```python
from build123d import *

# Parameters (mm, degrees)
F2_R = 8.554368
F3_R = 0.645964
F4_R = 0.880727
F5_R = 1.452178


with BuildPart() as f1:
    # F0 (on Front) → F1 (revolve)
    with BuildSketch(Plane.XZ):
        Polygon((-7.7875, 0), (0, 0), (0, 18.112501), (-0.9625, 18.112501), (-3.4125, 16.887501), (-6.0375, 12.1625), (-4.9875, 10.4125), (-6.0375, 10.2375), align=None)
    revolve(axis=Axis((0, 0, 9.056251), (0, 0, -1)))

    # F2
    f2_edges = [f1.edges().sort_by_distance(p)[0] for p in [
        (3.4125, 0, 16.887501),
    ]]
    fillet(f2_edges, radius=F2_R)

    # F3
    f3_edges = [f1.edges().sort_by_distance(p)[0] for p in [
        (6.0375, 0, 12.1625),
    ]]
    fillet(f3_edges, radius=F3_R)

    # F4
    f4_edges = [f1.edges().sort_by_distance(p)[0] for p in [
        (6.0375, 0, 10.2375),
    ]]
    fillet(f4_edges, radius=F4_R)

    # F5
    f5_edges = [f1.edges().sort_by_distance(p)[0] for p in [
        (7.7875, 0, 0),
    ]]
    fillet(f5_edges, radius=F5_R)


solid = f1.part
```
Check sheet for the modelled part. Datum: model origin and axes. Units: mm. Coordinates: 2 decimals unless noted, no trailing zeros. Loops run counter-clockwise (first coordinate to the right, second up) from the corner with the lowest first, then second, coordinate; pieces in that order, holes last.
1) Sectioned sample at A-A (z = 6). Record the boundary of the cut face in (x, y), and give its area (3 significant figures).
2) Gauge pin test, flat ends, axial feed: pin 1 (4 mm diameter, centred on x = -3.5, z = 9.5, fed in from +Y); pin 2 (5 mm diameter, centred on x = 1.5, z = 7, fed in from -Y); pin 3 (1.5 mm diameter, centred on x = 6, z = 9, fed in from +Y). Record the tip position at first contact, or that the pin passes through.
3) Sectioned sample at B-B (z = 9). Record the boundary of the cut face in (x, y), and give its area (3 significant figures).
4) Material ranges on probe 1 along X at (y, z) = (5.25, 1.5); probe 2 along Z at (x, y) = (-0.75, -2); probe 3 along X at (y, z) = (5.75, 5.25), recorded low to high.
Check sheet entries:
1. outline: circle Ø13.52 at (0, 0)
1. area: 144 mm2
2. pin 1: stops at y = 6.08
2. pin 2: stops at y = -6.96
2. pin 3: stops at y = 3.41
3. outline: circle Ø12.5 at (0, 0)
3. area: 123 mm2
4. probe 1: x = -5.38 to 5.38
4. probe 2: z = 0 to 17.42
4. probe 3: x = -3.8 to 3.8
